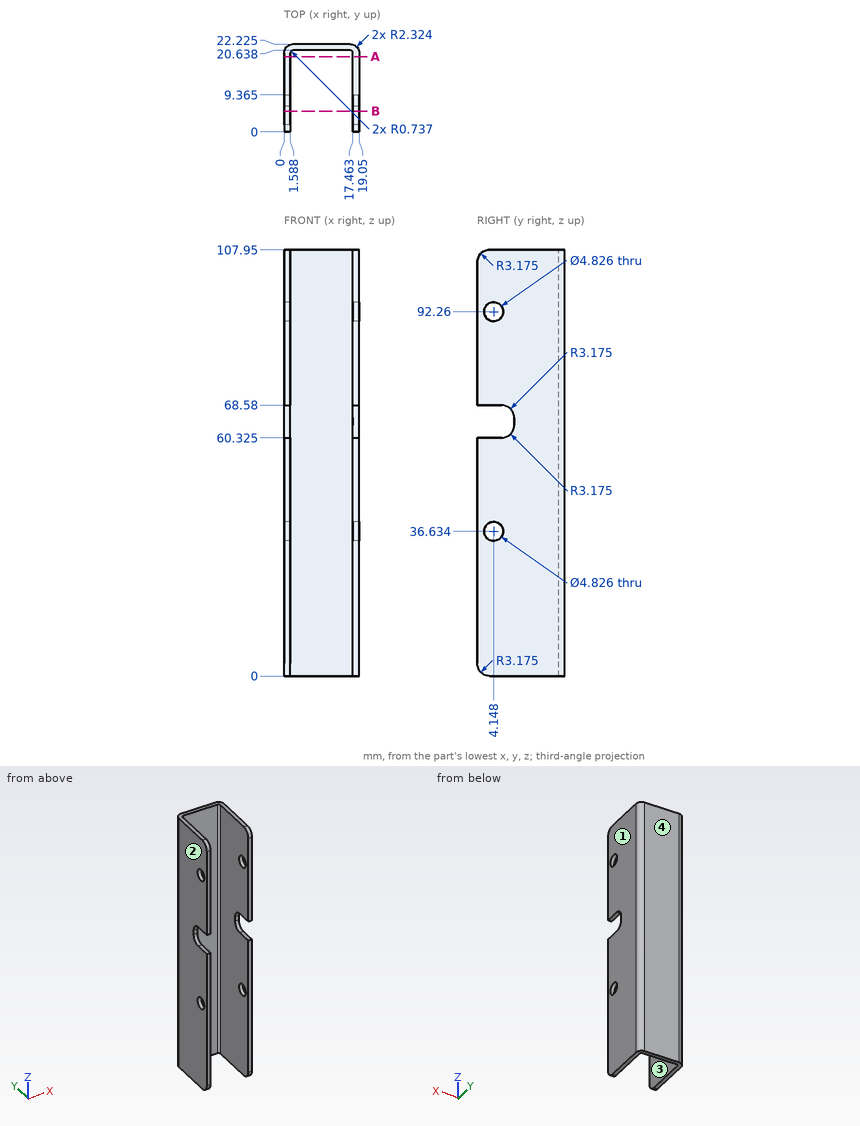
Geometry: see drawing. Coordinates: mm, zero at the bounding-box minimum. Round coordinates to 2 decimals unless told otherwise and drop trailing zeros. Loops run counter-clockwise (first coordinate to the right, second up) from the corner with the lowest first, then second, coordinate; pieces in that order, holes last. Notation, with made-up numbers: (43.5, 31) - (57.5, 31) arc R10 ccw to (57.5, 43) - close; hole circle Ø7 at (-25.5, 63.5). An arc over 180 degrees is marked (long way). Write item = value, one per line. Start each with the question number.
(1) Pin query (flat end, axial travel): pin 1 (1.3 mm diameter, centred on x = 18, z = 64.5, fed in from -Y) (1 decimal); pin 2 (3 mm diameter, centred on y = 4.15, z = 92.26, fed in from +X); pin 3 (1.3 mm diameter, centred on x = 18.5, y = 2, fed in from +Z). Return the tip coordinate at first contact, or that it passes through.
(2) Pull-direction query (X, two-part tool) for the marked faces 1, 2, 3 and 4; classes: +X half, -X half, draft (parallel to the pull), parting line (faces both ways), or undercut.
(3) Section query B-B, the plane y = 5.25. State how many separate pieces and enclosed holes the cut face has.
(4) Section query A-A, the plane y = 19. Output: boundary loops of the cut face in (x, z).
(5) Ray query, line 1 along X through (y, z) = (16.25, 65.5); line 2 along X through (y, z) = (20, 18.5) (1 decimal); line 3 along Y through (x, z) = (6, 55) (1 decimal). Return the intervals inside material, ascending. Write a range as from..to.
Conclusion:
q1.pin_1 = 9.4
q1.pin_2 = through
q1.pin_3 = 107.91
q2.face_1 = +X half
q2.face_2 = -X half
q2.face_3 = undercut
q2.face_4 = draft
q3.separate_pieces = 8
q3.enclosed_holes = 0
q4.outline = (0, 0) - (1.59, 0) - (1.59, 107.95) - (0, 107.95) - close; (17.46, 0) - (19.05, 0) - (19.05, 107.95) - (17.46, 107.95) - close
q5.line_1 = 0..1.59, 17.46..19.05
q5.line_2 = 0..1.6, 17.5..19
q5.line_3 = 20.6..22.2
